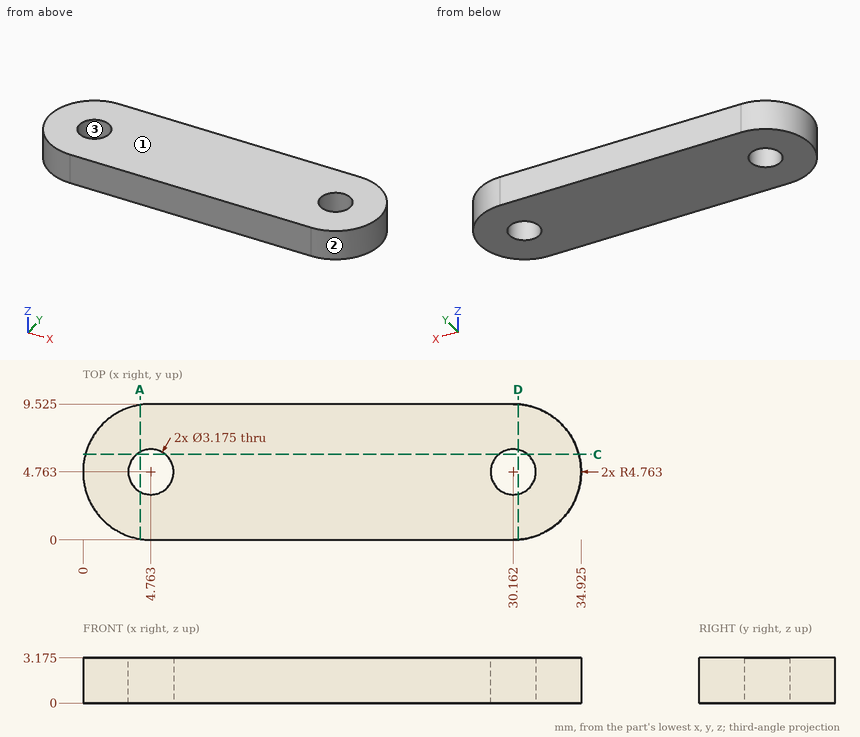
Print and shaded views of the part. All mm, measured from the part's lowest x, y and z. Coordinates: 2 decimals unless noted, no trailing zeros. Loops run counter-clockwise (first coordinate to the right, second up) from the corner with the lowest first, then second, coordinate; pieces in that order, holes last. Notation, with made-up numbers: (30.5, 7.5) - (75.5, 7.5) arc R36 cw to (75.5, 46.5) - close; hole circle Ø5 at (33.5, 64). An arc over 180 degrees is marked (long way). Write item = value, one per line. Start each with the question number.
Item 1: Wall check: probe 1 along X at (y, z) = (4, 2.65) (1 decimal); probe 2 along Y at (x, z) = (30.5, 1.4) (1 decimal); probe 3 along X at (y, z) = (7.25, 0.4) (1 decimal). Give the ranges that are in metal, low to high. Write a range as [from, to].
Item 2: Pull direction X, two halves, no side cores. Call the marked faces 1, 2 and 3: +X half, -X half, draft (parallel to the pull), parting line (faces both ways), or undercut.
Item 3: Saw through at A-A, the plane x = 4. List the corners of the cut face in (y, z) (1 decimal), then the cut area to 3 significant figures.
Item 4: Drop a flat-ended pin along its axis: pin 1 Ø1.5 at (y, z) = (2.5, 0.5) entering from +X. Give the stop position or say it passes through.
Item 5: Saw through at C-C, the plane y = 6. List the corners of the cut face in (x, z) (1 decimal).
Item 6: Saw through at D-D, the plane x = 30.5. List the corners of the cut face in (y, z) (1 decimal), then the cut area to 3 significant figures.
Answers:
q1.probe_1 = [0.1, 3.4], [6.2, 28.8], [31.6, 34.9]
q1.probe_2 = [0, 3.2], [6.3, 9.5]
q1.probe_3 = [0.7, 34.2]
q2.face_1 = draft
q2.face_2 = +X half
q2.face_3 = undercut
q3.outline = (0.1, 0) - (3.4, 0) - (3.4, 3.2) - (0.1, 3.2) - close; (6.2, 0) - (9.5, 0) - (9.5, 3.2) - (6.2, 3.2) - close
q3.area = 21.0 mm2
q4.pin_1 = 34.68
q5.outline = (0.2, 0) - (3.8, 0) - (3.8, 3.2) - (0.2, 3.2) - close; (5.8, 0) - (29.2, 0) - (29.2, 3.2) - (5.8, 3.2) - close; (31.2, 0) - (34.8, 0) - (34.8, 3.2) - (31.2, 3.2) - close
q6.outline = (0, 0) - (3.2, 0) - (3.2, 3.2) - (0, 3.2) - close; (6.3, 0) - (9.5, 0) - (9.5, 3.2) - (6.3, 3.2) - close
q6.area = 20.3 mm2
